Design review of the part shown in the three views and the two pictorial views. Dimensions are in mm from the part's minimum x, y and z. A direction names the side the tool comes from. Coordinates: 2 decimals unless noted, no trailing zeros. Loops run counter-clockwise (first coordinate to the right, second up) from the corner with the lowest first, then second, coordinate; pieces in that order, holes last. Notation, with made-up numbers: (74, 42) -> (112, 42) arc R11 cw to (112, 56) -> close; hole circle Ø5 at (29, 31). An arc over 180 degrees is marked (long way). Use CSV: the item, a comma, the result in double quotes.
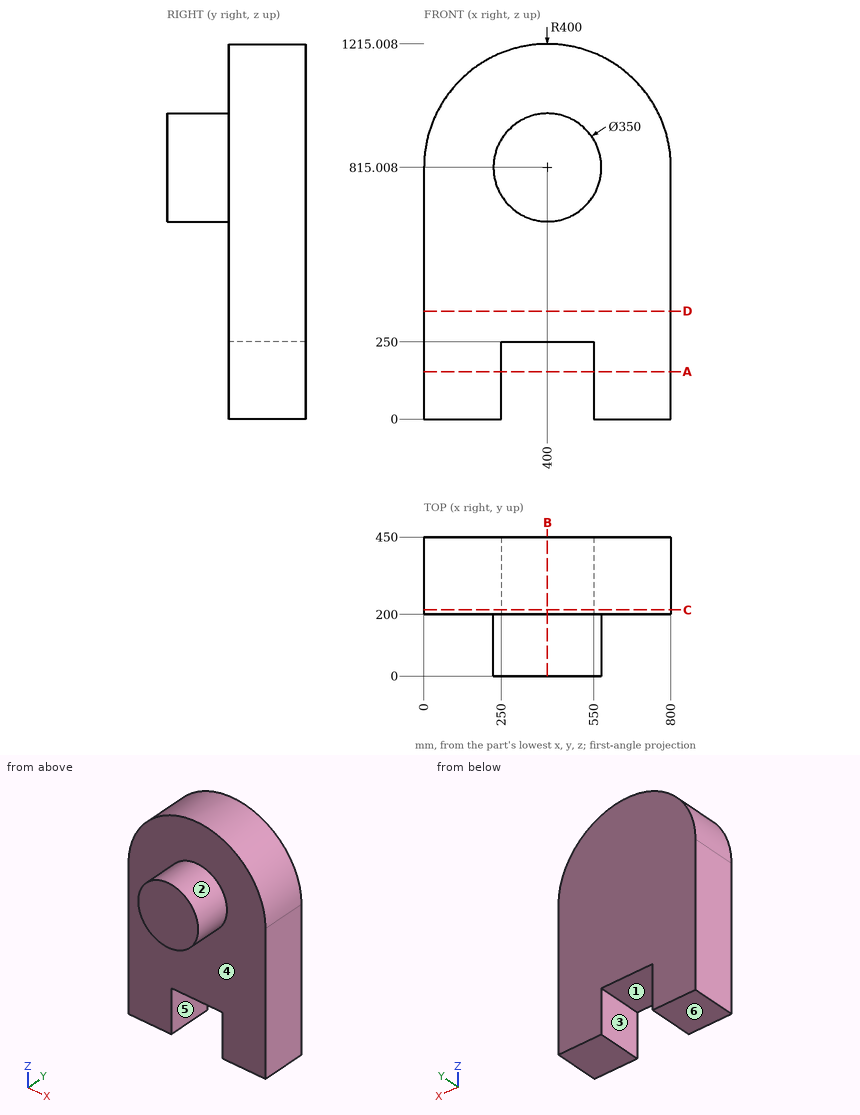
Item 1: Clearance check with flat-ended pins moving along their axes: pin 1 (1 mm diameter, centred on x = 474.5, y = 299, fed in from -Z); pin 2 (2 mm diameter, centred on x = 437, y = 144, fed in from -Z); pin 3 (1.5 mm diameter, centred on x = 633.5, y = 390, fed in from +Z). State where each tip first meets the part, or that it passes through.
Checked values:
pin 1,"z = 250"
pin 2,"z = 643.75"
pin 3,"z = 1140.32"
Item 2: Machinability: for the marked faces 5 and 6, which of the approach directions +Z, -Z, +X, -X, +Y, -Y give a long, thin tool a straight path to every point of the face, cutting with its end or side? Answer none if there is none.
Checked values:
face 5,"-Z, +Y, -Y"
face 6,"-Z, +X, -X, +Y, -Y"
Item 3: Add section C-C (y = 214.5). Give the boundary of the cut face in (x, z).
Checked values:
outline,"(0, 0) -> (250, 0) -> (250, 250) -> (550, 250) -> (550, 0) -> (800, 0) -> (800, 815.01) arc R400 ccw to (0, 815.01) -> close"
Item 4: Add section A-A (z = 154). Give the boundary of the cut face in (x, y), then the cut area to 3 significant figures.
Checked values:
outline,"(0, 200) -> (250, 200) -> (250, 450) -> (0, 450) -> close; (550, 200) -> (800, 200) -> (800, 450) -> (550, 450) -> close"
area,"125,000 mm^2"
Item 5: Add section D-D (z = 350). Give the boundary of the cut face in (x, y), then the cut area to 3 significant figures.
Checked values:
outline,"(0, 200) -> (800, 200) -> (800, 450) -> (0, 450) -> close"
area,"200,000 mm^2"
Item 6: To check wall thickness, follow line 1 along Y through (x, z) = (54, 190); line 2 along X through (y, z) = (245, 227); line 3 along X through (y, z) = (199.5, 813.5). State the ranges of each line that lie inside material, in increasing order.
Checked values:
line 1,"200 to 450"
line 2,"0 to 250, 550 to 800"
line 3,"225.01 to 574.99"
Item 7: Add section B-B (x = 400). Give the boundary of the cut face in (y, z), then the cut area to 3 significant figures.
Checked values:
outline,"(0, 640.01) -> (200, 640.01) -> (200, 250) -> (450, 250) -> (450, 1215.01) -> (200, 1215.01) -> (200, 990.01) -> (0, 990.01) -> close"
area,"311,000 mm^2"
Item 8: Draft analysis for pull direction X (two halves, no side actions). For the marked faces 1, 2, 3 and 4, state which applies: pulls with the +X half, pulls with the -X half, needs draft (parallel to the pull), parting line crosses it, or undercut.
Checked values:
face 1,"undercut"
face 2,"parting line crosses it"
face 3,"undercut"
face 4,"needs draft"
